Could you check a few things on this model? Use its own coordinates, in mm. A direction names the side the tool comes from. Round coordinates to 2 decimals unless told otherwise and drop trailing zeros. Order: outer loops, then holes, each group sorted by start corner. A loop starts at its lowest first (then second) coordinate and runs counter-clockwise, first axis right, second up. Notation, with made-up numbers: (77.25, 78.5) -> (90.25, 78.5) arc R19 ccw to (90.25, 98.5) -> close; hole circle Ø10 at (79, 11). An arc over 180 degrees is marked (long way). One line per question, with ' | ' between items.
```python
from build123d import *

# Parameters (mm, degrees)
F1_DEPTH      = 25
F1_DEPTH_BACK = 25
F2_SIZE       = 5
F3_R          = 4.05
F4_DEPTH      = 20
F6_DEPTH      = 2
F7_SIZE       = 1


with BuildPart() as f1:
    # F0 (on Top) → F1 (new body, two sides)
    with BuildSketch(Plane.XY) as f1_sk:
        with BuildLine():
            Line((42.4409423598, 91.1082738708), (11.7302642411, 60.3975957521))
            ThreePointArc((11.7302642411, 60.3975957521), (3.0593541881, 47.4206617993), (0.0145354886, 32.1133245047))
            Line((0.0145354886, 32.1133245047), (0.0145354886, 0.1133245047))
            Line((0.0145354886, 0.1133245047), (20.0145354886, 0.1133245047))
            Line((20.0145354886, 0.1133245047), (20.0145354886, 32.1133245047))
            ThreePointArc((20.0145354886, 32.1133245047), (21.5369448383, 39.766993152), (25.8723998648, 46.2554601284))
            Line((25.8723998648, 46.2554601284), (56.5830779835, 76.9661382471))
            ThreePointArc((56.5830779835, 76.9661382471), (56.5830779835, 91.1082738708), (42.4409423598, 91.1082738708))
        make_face()
    extrude(amount=F1_DEPTH)
    extrude(f1_sk.sketch, amount=-F1_DEPTH_BACK)

    # F2
    f2_edges = [f1.edges().sort_by_distance(p)[0] for p in [
        (0.014535, 16.113325, 25),
        (3.059354, 47.420662, 25),
        (27.085603, 75.752935, 25),
        (56.583078, 91.108274, 25),
        (41.227739, 61.610799, 25),
        (21.536945, 39.766993, 25),
        (20.014535, 16.113325, 25),
        (41.227739, 61.610799, -25),
        (56.583078, 91.108274, -25),
        (27.085603, 75.752935, -25),
        (3.059354, 47.420662, -25),
        (0.014535, 16.113325, -25),
        (21.536945, 39.766993, -25),
        (20.014535, 16.113325, -25),
    ]]
    chamfer(f2_edges, length=F2_SIZE)

    # F3 (on face) → F4 (cut)
    with BuildSketch(Plane.XZ.offset(-0.1133245047)):
        with Locations((10.0145354886, 10)):
            Circle(F3_R)
        with Locations((10.0145354886, -10)):
            Circle(F3_R)
    extrude(amount=-F4_DEPTH, mode=Mode.SUBTRACT)

    # F5 (on face) → F6 (cut)
    with BuildSketch(Plane.XY.offset(25)):
        with BuildLine():
            Line((12.0145354886, 12.6133245047), (20.0145354886, 12.6133245047))
            Line((20.0145354886, 12.6133245047), (20.0145354886, 19.6133245047))
            Line((20.0145354886, 19.6133245047), (12.0145354886, 19.6133245047))
            ThreePointArc((12.0145354886, 19.6133245047), (10.6003219262, 19.027538067), (10.0145354886, 17.6133245047))
            Line((10.0145354886, 17.6133245047), (10.0145354886, 14.6133245047))
            ThreePointArc((10.0145354886, 14.6133245047), (10.6003219262, 13.1991109423), (12.0145354886, 12.6133245047))
        make_face()
    extrude(amount=-F6_DEPTH, mode=Mode.SUBTRACT)

    # F7
    f7_edges = [f1.edges().sort_by_distance(p)[0] for p in [
        (10.600322, 19.027538, 25),
        (10.014535, 16.113325, 25),
        (10.600322, 13.199111, 25),
        (13.514535, 12.613325, 25),
        (16.014535, 12.613325, 24),
        (13.514535, 19.613325, 25),
        (16.014535, 19.613325, 24),
    ]]
    chamfer(f7_edges, length=F7_SIZE)


solid = f1.part
```
1. On a 3-axis mill with a long thin cutter (end or side, diameter ignored), from which of +Z, -Z, +X, -X, +Y, -Y can I reach the whole of each face in a straight line? I mean faces 4 (the face through (10.616, 19.043, 23.507)), 5 (the face through (29.093, 74.175, -22.535)), 6 (the face through (27.3, 75.97, 0.28)), 7 (the face through (17.48, 15.889, 22.535)), 8 (the face through (11.883, 9.973, 6.407)). Say none if no direction works.
From the geometry:
face 4: +Z, +X | face 5: -Z, -X, +Y | face 6: +Z, -Z, -X, +Y | face 7: +Z, +X, -Y | face 8: -Y
2. I want a section at C-C on z = 7.5. List the corners of the cut face in (x, y) for me.
From the geometry:
outline: (0.01, 0.11) -> (6.83, 0.11) -> (6.83, 20.11) -> (13.2, 20.11) -> (13.2, 0.11) -> (20.01, 0.11) -> (20.01, 32.11) arc R20 cw to (25.87, 46.26) -> (56.58, 76.97) arc R10 ccw to (42.44, 91.11) -> (11.73, 60.4) arc R40 ccw to (0.01, 32.11) -> close
3. I'm going to push flat-ended pins straight in: pin 1 (2 mm diameter, centred on x = 13, y = 16.5, fed in from +Z); pin 2 (1.5 mm diameter, centred on x = 15, y = 58.5, fed in from +Z); pin 3 (0.5 mm diameter, centred on y = 16, z = 23.5, fed in from +X). Where does each tip first touch, or does it pass through?
From the geometry:
pin 1: stops at z = 23 | pin 2: stops at z = 24.4 | pin 3: stops at x = 10.01
4. I want a section at A-A on z = -10. List the corners of the cut face in (x, y) for me.
From the geometry:
outline: (0.01, 0.11) -> (5.96, 0.11) -> (5.96, 20.11) -> (14.06, 20.11) -> (14.06, 0.11) -> (20.01, 0.11) -> (20.01, 32.11) arc R20 cw to (25.87, 46.26) -> (56.58, 76.97) arc R10 ccw to (42.44, 91.11) -> (11.73, 60.4) arc R40 ccw to (0.01, 32.11) -> close
5. I want a section at B-B on y = 70.5. List the corners of the cut face in (x, z) for me.
From the geometry:
outline: (21.83, -20) -> (28.9, -25) -> (43.05, -25) -> (50.12, -20) -> (50.12, 20) -> (43.05, 25) -> (28.9, 25) -> (21.83, 20) -> close
6. I need wall thicknesses on probe 1 along X at (y, z) = (33, 16.5); probe 2 along X at (y, z) = (35, 7); probe 3 along Z at (x, y) = (24, 67.5). Which ranges of each line are inside material? Lowest first, please.
From the geometry:
probe 1: x = 0.02 to 20.03 | probe 2: x = 0.12 to 20.22 | probe 3: z = -23.65 to 23.65
7. If we mould it in two halves opening along Y, with no side actions, what happens to faces 1 (the face through (10.349, 19.316, 24.382)), 2 (the face through (2.55, 16.337, 22.535)), 3 (the face through (5.993, 46.425, 23.091))? For each: pulls with the +Y half, pulls with the -Y half, needs draft (parallel to the pull), parting line crosses it, or undercut.
From the geometry:
face 1: undercut | face 2: needs draft | face 3: pulls with the +Y half
